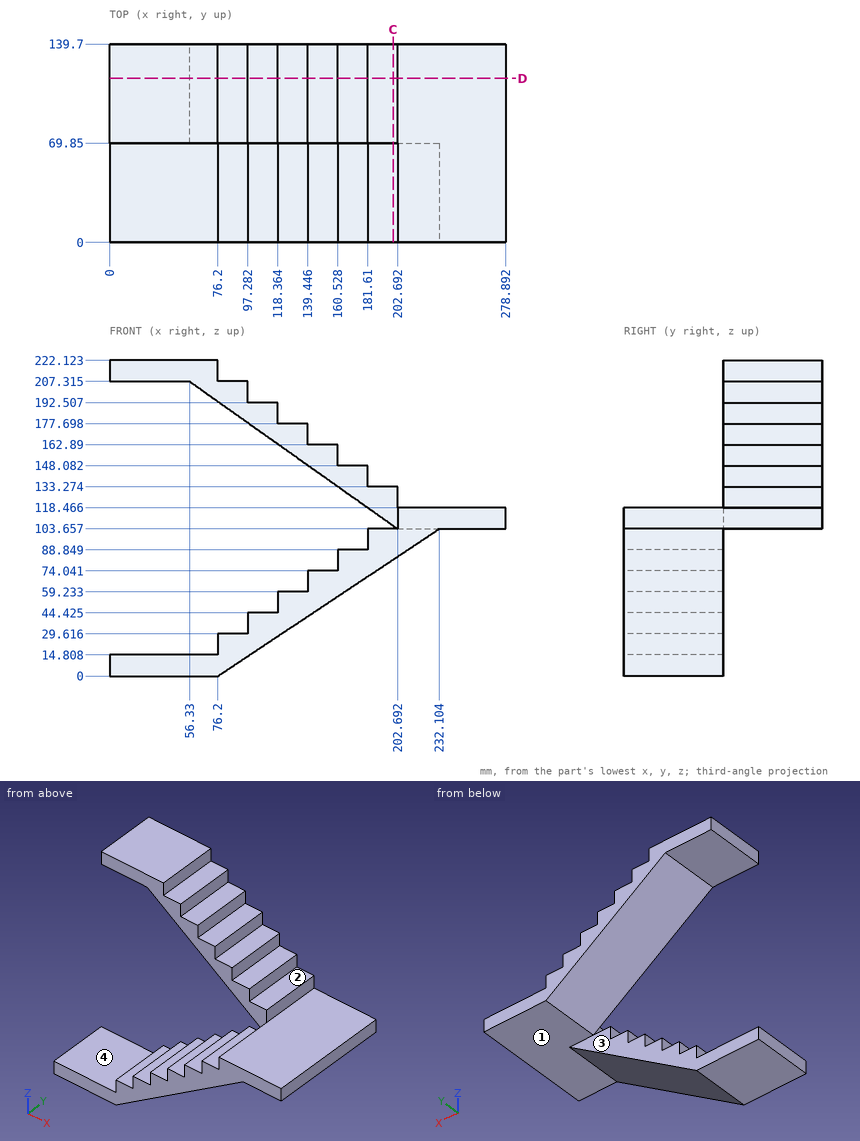
Geometry: see drawing. Coordinates: mm, zero at the bounding-box minimum. A direction names the side the tool comes from. Round coordinates to 2 decimals unless told otherwise and drop trailing zeros. Write each loop counter-clockwise with the first axis right and the second up, starting at its lowest first coordinate (ties: lowest second). Pieces come first, ordered by that corner, then holes. Notation, with made-up numbers: (59, -13.5) - (108, -13.5) arc R4 ccw to (108, -9.5) - close; hole circle Ø9 at (46.25, 25). An arc over 180 degrees is marked (long way). Use CSV: the item, a comma, the result in double quotes. Start each with the question number.
(1) Set-up query: the marked faces 1, 2, 3 and 4. Return all of +Z, -Z, +X, -X, +Y, -Y with unobstructed straight access to the full face (end or side cutting, diameter ignored); none if empty.
(2) First-contact query: pin 1 Ø6.5 at (x, y) = (83.5, 25.5) entering from +Z; pin 2 Ø1 at (x, y) = (32, 30) entering from +Z; pin 3 Ø1.5 at (x, y) = (93.5, 22) entering from -Z. Flat tips, straight axial feed; report the tip coordinate or a pass-through.
(3) Material intervals for probe 1 along Z at (x, y) = (255, 71.5) (1 decimal); probe 2 along Z at (x, y) = (20, 86.5) (1 decimal); probe 3 along X at (y, z) = (65.5, 110), sorted ascending. Write a range as [from, to].
(4) Cut plane C-C, the plane x = 199.5. Return loops of the section in (y, z).
(5) Cut plane D-D, the plane y = 115.5. Return loops of the section in (x, z) (1 decimal), and give its area (3 significant figures).
Geometry says:
1,face 1,"-Z, +X, +Y"
1,face 2,"+Z, +X, +Y, -Y"
1,face 3,"-Z, +X, -X, +Y"
1,face 4,"+Z, -X, +Y, -Y"
2,pin 1,"z = 29.62"
2,pin 2,"z = 14.81"
2,pin 3,"z = 11"
3,probe 1,"[103.7, 118.5]"
3,probe 2,"[207.3, 222.1]"
3,probe 3,"[202.69, 278.89]"
4,outline,"(0, 81.98) - (69.85, 81.98) - (69.85, 103.66) - (0, 103.66) - close; (69.85, 105.92) - (139.7, 105.92) - (139.7, 133.27) - (69.85, 133.27) - close"
5,outline,"(0, 207.3) - (56.3, 207.3) - (202.7, 103.7) - (278.9, 103.7) - (278.9, 118.5) - (202.7, 118.5) - (202.7, 133.3) - (181.6, 133.3) - (181.6, 148.1) - (160.5, 148.1) - (160.5, 162.9) - (139.4, 162.9) - (139.4, 177.7) - (118.4, 177.7) - (118.4, 192.5) - (97.3, 192.5) - (97.3, 207.3) - (76.2, 207.3) - (76.2, 222.1) - (0, 222.1) - close"
5,area,"5,160 mm²"
